The listing builds one solid part. Answer for the finished solid, in the listing's coordinates (mm). Give positions to 0.01 mm unless a question says otherwise; leave off trailing zeros. Write each loop counter-clockwise with the first axis right and the second up, starting at its lowest first coordinate (ties: lowest second). Pieces come first, ordered by that corner, then holes.
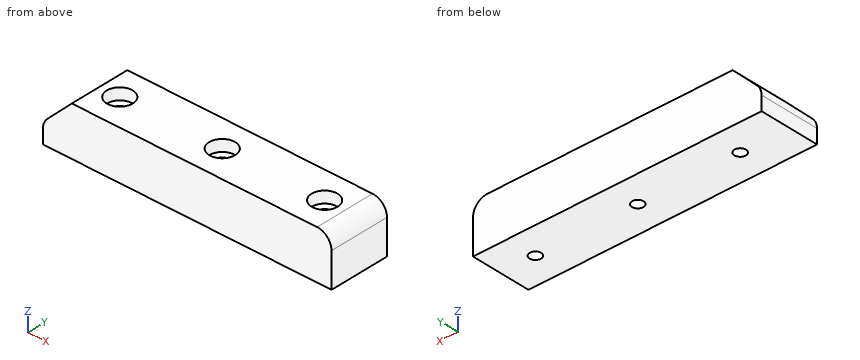
```python
from build123d import *

# Parameters (mm, degrees)
F1_DEPTH = 21
F2_R     = 5
F3_R     = 5
F5_DEPTH = 25
F6_R     = 4.5
F7_DEPTH = 4


with BuildPart() as f1:
    # F0 (on Front) → F1 (new body)
    with BuildSketch(Plane.XZ):
        Polygon((-3, 7), (-3, 0), (97, 0), (97, 17), (7, 17), align=None)
    extrude(amount=F1_DEPTH)

    # F2
    f2_edges = [f1.edges().sort_by_distance(p)[0] for p in [
        (97, -10.5, 17),
    ]]
    fillet(f2_edges, radius=F2_R)

    # F3
    f3_edges = [f1.edges().sort_by_distance(p)[0] for p in [
        (-3, -10.5, 7),
    ]]
    fillet(f3_edges, radius=F3_R)

    # F4 (on face) → F5 (cut)
    with BuildSketch(Plane.XY.offset(17)):
        with BuildLine():
            ThreePointArc((87, -10.5), (85, -8.5), (83, -10.5))
            Line((83, -10.5), (87, -10.5))
        make_face()
        with BuildLine():
            Line((87, -10.5), (83, -10.5))
            ThreePointArc((83, -10.5), (85, -12.5), (87, -10.5))
        make_face()
        with BuildLine():
            ThreePointArc((51.5, -10.5), (49.5, -8.5), (47.5, -10.5))
            Line((47.5, -10.5), (51.5, -10.5))
        make_face()
        with BuildLine():
            Line((51.5, -10.5), (47.5, -10.5))
            ThreePointArc((47.5, -10.5), (49.5, -12.5), (51.5, -10.5))
        make_face()
        with BuildLine():
            ThreePointArc((12, -10.5), (14, -12.5), (16, -10.5))
            Line((16, -10.5), (12, -10.5))
        make_face()
        with BuildLine():
            Line((12, -10.5), (16, -10.5))
            ThreePointArc((16, -10.5), (14, -8.5), (12, -10.5))
        make_face()
    extrude(amount=-F5_DEPTH, mode=Mode.SUBTRACT)

    # F6 (on face) → F7 (cut)
    with BuildSketch(Plane.XY.offset(17)):
        with Locations((14, -10.5)):
            Circle(F6_R)
        with Locations((49.5, -10.5)):
            Circle(F6_R)
        with Locations((85, -10.5)):
            Circle(F6_R)
    extrude(amount=-F7_DEPTH, mode=Mode.SUBTRACT)


solid = f1.part
```
Item 1: A cutting plane is placed at A-A, the plane x = 14. Give the vertices of the cut face in (y, z).
Conclusion:
outline: (-21, 0) - (-12.5, 0) - (-12.5, 13) - (-15, 13) - (-15, 17) - (-21, 17) - close; (-8.5, 0) - (0, 0) - (0, 17) - (-6, 17) - (-6, 13) - (-8.5, 13) - close
Item 2: Consider probe 1 along Y at (x, z) = (49.5, 13.9); probe 2 along X at (y, z) = (-9, 6.75); probe 3 along Y at (x, z) = (14, 4). Determine where each line is inside the solid, lowest interval first.
Conclusion:
probe 1: y = -21 to -15, -6 to 0
probe 2: x = -2.66 to 12.68, 15.32 to 48.18, 50.82 to 83.68, 86.32 to 97
probe 3: y = -21 to -12.5, -8.5 to 0
Item 3: A cutting plane is placed at B-B, the plane y = -10.5. Count the separate pieces of the cut face and the enclosed holes in it, plus the area to 3 significant figures.
Conclusion:
separate pieces: 4
enclosed holes: 0
area: 1,380 mm2
Item 4: A cutting plane is placed at C-C, the plane z = 10. Give the vertices of the cut face in (x, y).
Conclusion:
outline: (0, -21) - (97, -21) - (97, 0) - (0, 0) - close; hole circle Ø4 at (14, -10.5); hole circle Ø4 at (49.5, -10.5); hole circle Ø4 at (85, -10.5)
Item 5: Each of these flat-tipped pins is pushed along its axis until it touches: P1, Ø1.5, axis at y = -17, z = 6, coming from the -X side; P2, Ø4.5, axis at x = 85, y = -10.5, coming from the +Z side. Where does it stop, or does it pass through?
Conclusion:
P1: stops at x = -2.99
P2: stops at z = 13
Item 6: A cutting plane is placed at D-D, the plane y = -1.25. Give the vertices of the cut face in (x, z), plus the area to 3 significant figures.
Conclusion:
outline: (-3, 0) - (97, 0) - (97, 12) arc R5 ccw to (92, 17) - (7, 17) - (-1.54, 8.46) arc R5 ccw to (-3, 4.93) - close
area: 1,640 mm2
